Autodesk Inventor part; units mm, degrees
ref_plane "YZ Plane" through (0, 0, 0) normal (1, 0, 0) x (0, 1, 0)
ref_plane "XZ Plane" through (0, 0, 0) normal (0, 1, 0) x (-1, 0, 0)
ref_plane "XY Plane" through (0, 0, 0) normal (0, 0, 1) x (1, 0, 0)
sketch "main" plane through (0, 0, 0) normal (0, 0, 1) x (1, 0, 0)
  circle A0 centre (-24.2926, 27.4457) radius 2.1844
  circle A1 centre (-24.2926, -48.7543) radius 2.1844
  circle A2 centre (26.5074, 27.4457) radius 2.1844
  arc A3 (-30.6426, -48.7543) -> (-19.0091, -52.2766) centre (-24.2926, -48.7543) ccw
  arc A4 (31.7909, 23.9234) -> (26.5074, 33.7957) centre (26.5074, 27.4457) ccw
  arc A5 (-24.2926, 33.7957) -> (-30.6426, 27.4457) centre (-24.2926, 27.4457) ccw
  line L0 (-30.6426, -48.7543) -> (-30.6426, 27.4457)
  line L1 (-24.2926, 33.7957) -> (26.5074, 33.7957)
  line L2 (31.7909, 23.9234) -> (-19.0091, -52.2766)
  line L3 (-16.3551, -22.5385) -> (11.6761, 19.5082)
  line L4 (11.6761, 19.5082) -> (-16.3551, 19.5082)
  line L5 (-16.3551, 19.5082) -> (-16.3551, -22.5385)
  circle A6 centre (-24.2926, 14.7457) radius 2.1844
  point P0 (-7.9432, 11.0963)
  dimension "d0" = 12.7
  dimension "d1" = 12.7
  dimension "d2" = 12.7
  dimension "d3" = 14.2875
  dimension "d6" = 4.3688
  dimension "d7" = 76.2
  dimension "d8" = 0
sketch "Sketch1" plane through (0, 0, 0) normal (0, 1, 0) x (-1, 0, 0)
  circle A0 centre (0, 0) radius 2.1844
  circle A1 centre (0, -76.2) radius 2.1844
  circle A2 centre (50.8, 0) radius 2.1844
  arc A3 (-6.35, -76.2) -> (5.2835, -79.7223) centre (0, -76.2) ccw
  arc A4 (56.0835, -3.5223) -> (50.8, 6.35) centre (50.8, 0) ccw
  arc A5 (0, 6.35) -> (-6.35, 0) centre (0, 0) ccw
  line L0 (-6.35, -76.2) -> (-6.35, 0)
  line L1 (0, 6.35) -> (50.8, 6.35)
  line L2 (56.0835, -3.5223) -> (5.2835, -79.7223)
  line L3 (7.9375, -49.9842) -> (35.9686, -7.9375)
  line L4 (35.9686, -7.9375) -> (7.9375, -7.9375)
  line L5 (7.9375, -7.9375) -> (7.9375, -49.9842)
  circle A6 centre (0, -12.7) radius 2.1844
extrude "Extrusion1" add sketch "Sketch1" along normal blind 1.5875
properties part number "Triangle Gusset" material "Acetal Resin, White"
Could you check a few things on this model? Use its own coordinates, in mm. Coordinates: 2 decimals unless noted, no trailing zeros. Order: outer loops, then holes, each group sorted by start corner. A loop starts at its lowest first (then second) coordinate and runs counter-clockwise, first axis right, second up. Notation, with made-up numbers: (78.5, 87.5) -> (91.5, 87.5) arc R11 cw to (91.5, 94.5) -> close; hole circle Ø5 at (-22, 37). An arc over 180 degrees is marked (long way). One line per item, written item: value. Start each with the question number.
1) Imagine slicing it at B-B on x = -23. List the corners of the cut face in (y, z) for me.
2) If I drill on L1, parallel to Z at x = 0, y = 1; L2, parallel to X at y = 1.3, z = -8; L3, parallel to X at y = 0.7, z = 1.5, over which ranges is the centre line in solid material (lowest first)? Write a range as [from, to].
3) I'm going to push flat-ended pins straight in: pin 1 (0.8 mm diameter, centred on x = -21.5, y = 0.5, fed in from -Z); pin 2 (0.8 mm diameter, centred on y = 0.5, z = -27, fed in from -X). Where does each tip first touch, or does it pass through?
4) Imagine slicing it at C-C on z = -12.7. List the corners of the cut face in (x, y) for me.
5) Imagine slicing it at D-D on z = -23.5. List the corners of the cut face in (x, y) for me, plus the area to 3 significant figures.
6) We'd pull the mould along Z, two halves only. Please class faces 1 (the cylindrical face through (4.54, 0.78, 4.44)), 2 (the flat face through (-21.757, 0.783, -29.255)), 3 (the cylindrical face through (-52.818, 0.783, 0.837)), 4 (the cylindrical face through (-56.353, 0.783, 3.081)): +Z half, -Z half, draft (parallel to the pull), parting line (faces both ways), or undercut.
7) Imagine slicing it at A-A on y = 0.45. List the corners of the cut face in (x, z) for me.
Answer list:
1. outline: (0, -53.15) -> (1.59, -53.15) -> (1.59, -27.39) -> (0, -27.39) -> close; (0, -7.94) -> (1.59, -7.94) -> (1.59, 6.35) -> (0, 6.35) -> close
2. L1: z = [-82.55, -78.38], [-74.02, -14.88], [-10.52, -2.18], [2.18, 6.35]
2. L2: x = [-53.1, -35.93], [-7.94, 6.35]
2. L3: x = [-56.97, -52.39], [-49.21, -1.59], [1.59, 6.17]
3. pin 1: stops at z = -56
3. pin 2: stops at x = -40.7
4. outline: (-49.97, 0) -> (-32.79, 0) -> (-32.79, 1.59) -> (-49.97, 1.59) -> close; (-7.94, 0) -> (-2.18, 0) -> (-2.18, 1.59) -> (-7.94, 1.59) -> close; (2.18, 0) -> (6.35, 0) -> (6.35, 1.59) -> (2.18, 1.59) -> close
5. outline: (-42.77, 0) -> (-25.59, 0) -> (-25.59, 1.59) -> (-42.77, 1.59) -> close; (-7.94, 0) -> (6.35, 0) -> (6.35, 1.59) -> (-7.94, 1.59) -> close
5. area: 49.9 mm2
6. face 1: +Z half
6. face 2: undercut
6. face 3: undercut
6. face 4: parting line
7. outline: (-56.08, -3.52) -> (-5.28, -79.72) arc R6.35 ccw to (6.35, -76.2) -> (6.35, 0) arc R6.35 ccw to (0, 6.35) -> (-50.8, 6.35) arc R6.35 ccw to start; hole circle Ø4.37 at (-50.8, 0); hole (-35.97, -7.94) -> (-7.94, -49.98) -> (-7.94, -7.94) -> close; hole circle Ø4.37 at (0, -76.2); hole circle Ø4.37 at (0, -12.7); hole circle Ø4.37 at (0, 0)
